Input: part model. Units: mm. Frame: model coordinates. A direction names the side the tool comes from. Round coordinates to 2 decimals unless told otherwise and drop trailing zeros. Order: outer loops, then holes, each group sorted by start corner. A loop starts at its lowest first (then second) coordinate and runs counter-clockwise, first axis right, second up. Notation, with made-up numbers: (68.5, 5.25) -> (114.5, 5.25) arc R24 ccw to (114.5, 16.25) -> close; hole circle Ø3 at (5.5, 35). An arc over 180 degrees is marked (long way). Use a Markdown table: item, result.
from build123d import *

# Parameters (mm, degrees)
SKETCH1_R           = 2.5
SKETCH1_R_2         = 1.3
BOSS_EXTRUDE1_DEPTH = 5
SKETCH2_W           = 40
SKETCH2_H           = 25
BOSS_EXTRUDE2_DEPTH = 10
SKETCH3_W           = 23
SKETCH3_H           = 13
CUT_EXTRUDE1_DEPTH  = 8
SKETCH3_3_R         = 1.05
CUT_EXTRUDE2_DEPTH  = 8
SKETCH3_4_W         = 23
SKETCH3_4_H         = 13
CUT_EXTRUDE3_DEPTH  = 11
FILLET1_R           = 10
CUT_EXTRUDE4_DEPTH  = 41


with BuildPart() as part:
    # Sketch1 → Boss-Extrude1 (new body)
    with BuildSketch(Plane(origin=(0, 0, 0), x_dir=(1, 0, 0), z_dir=(0, 1, 0))):
        with BuildLine():
            Line((0, 15), (25, 15))
            Line((25, 15), (25, -15))
            Line((25, -15), (0, -15))
            ThreePointArc((0, -15), (-15, 0), (0, 15))
        make_face()
        Circle(SKETCH1_R, mode=Mode.SUBTRACT)
        with Locations((0, -4.5)):
            Circle(SKETCH1_R_2, mode=Mode.SUBTRACT)
        with Locations((0, 4.5)):
            Circle(SKETCH1_R_2, mode=Mode.SUBTRACT)
    extrude(amount=BOSS_EXTRUDE1_DEPTH)

    # Sketch2 → Boss-Extrude2 (add)
    with BuildSketch(Plane(origin=(25, 0, 0), x_dir=(0, 0, -1), z_dir=(1, 0, 0))):
        with Locations((5, 12.5)):
            Rectangle(SKETCH2_W, SKETCH2_H)
    extrude(amount=BOSS_EXTRUDE2_DEPTH)

    # Sketch3 → Cut-Extrude1 (cut)
    with BuildSketch(Plane(origin=(25, 0, 0), x_dir=(0, 0, -1), z_dir=(1, 0, 0))):
        with Locations((5, 13)):
            Rectangle(SKETCH3_W, SKETCH3_H)
    extrude(amount=CUT_EXTRUDE1_DEPTH, mode=Mode.SUBTRACT)

    # Sketch3<3> → Cut-Extrude2 (cut)
    with BuildSketch(Plane(origin=(25, 0, 0), x_dir=(0, 0, -1), z_dir=(1, 0, 0))):
        with Locations((-9, 13)):
            Circle(SKETCH3_3_R)
        with Locations((19, 13)):
            Circle(SKETCH3_3_R)
    extrude(amount=CUT_EXTRUDE2_DEPTH, mode=Mode.SUBTRACT)

    # Sketch3<4> → Cut-Extrude3 (cut, through all)
    with BuildSketch(Plane(origin=(25, 0, 0), x_dir=(0, 0, -1), z_dir=(1, 0, 0))):
        with Locations((5, 13)):
            Rectangle(SKETCH3_4_W, SKETCH3_4_H)
    extrude(amount=CUT_EXTRUDE3_DEPTH, mode=Mode.SUBTRACT)

    # Fillet1
    fillet1_edges = [part.edges().sort_by_distance(p)[0] for p in [
        (30, 0, -25),
        (30, 25, -25),
        (30, 25, 15),
    ]]
    fillet(fillet1_edges, radius=FILLET1_R)

    # Sketch4 → Cut-Extrude4 (cut, through all)
    with BuildSketch(Plane.XY.offset(15)):
        Polygon((7, 0), (4, 3), (-4, 3), (-7, 0), align=None)
    extrude(amount=-CUT_EXTRUDE4_DEPTH, mode=Mode.SUBTRACT)


solid = part.part
1) Cut plane C-C on x = -9. Return loops of the section in (y, z).
Results found:
| item | result |
|---|---|
| outline | (0, -12) -> (5, -12) -> (5, 12) -> (0, 12) -> close |
2) Cut plane A-A on z = 0. Return loops of the section in (x, y), and give its area (3 significant figures).
Results found:
| item | result |
|---|---|
| outline | (-15, 0) -> (-7, 0) -> (-4, 3) -> (-2.5, 3) -> (-2.5, 5) -> (-15, 5) -> close; (2.5, 3) -> (4, 3) -> (7, 0) -> (35, 0) -> (35, 6.5) -> (25, 6.5) -> (25, 5) -> (2.5, 5) -> close; (25, 19.5) -> (35, 19.5) -> (35, 25) -> (25, 25) -> close |
| area | 277 mm² |
3) Line query: L1, parallel to Z at x = 0, y = 3.7; L2, parallel to Y at x = 11, z = 0.5; L3, parallel to X at y = 5.25, z = -13. Output: solid intervals per line, ascending. Write a range as [from, to].
Results found:
| item | result |
|---|---|
| L1 | z = [-15, -5.8], [-3.2, -2.5], [2.5, 3.2], [5.8, 15] |
| L2 | y = [0, 5] |
| L3 | x = [25, 35] |
4) Cut plane B-B on y = 13. Return loops of the section in (x, z).
Results found:
| item | result |
|---|---|
| outline | (25, -25) -> (35, -25) -> (35, -16.5) -> (25, -16.5) -> (25, -17.95) -> (33, -17.95) -> (33, -20.05) -> (25, -20.05) -> close; (25, 6.5) -> (35, 6.5) -> (35, 15) -> (25, 15) -> (25, 10.05) -> (33, 10.05) -> (33, 7.95) -> (25, 7.95) -> close |
5) Cut plane D-D on z = -19. Return loops of the section in (x, y), and give its area (3 significant figures).
Results found:
| item | result |
|---|---|
| outline | (25, 0.83) -> (35, 0.83) -> (35, 24.17) -> (25, 24.17) -> (25, 14.05) -> (33, 14.05) -> (33, 11.95) -> (25, 11.95) -> close |
| area | 217 mm² |
6) Set-up query: faces 5 (the flat face through (5, 5, 0)), 6 (the flat face through (-5, 2, 0)), 7 (the flat face through (30, 6.5, -5)), 8 (the flat face through (33, 13, 9)). Return all of +Z, -Z, +X, -X, +Y, -Y with unobstructed straight access to the full face (end or side cutting, diameter ignored); none if empty.
Results found:
| item | result |
|---|---|
| face 5 | +Z, -Z, -X, +Y |
| face 6 | +Z, -Z, -Y |
| face 7 | +X, -X |
| face 8 | -X |
7) Pull-direction query (Z, two-part tool) for faces 1 (the cylindrical face through (28.94, 13.05, -17.95)), 2 (the flat face through (21, 0, 0)), 3 (the cylindrical face through (-0.28, 3.99, -3.23)), 4 (the flat face through (12, 2, -15)); classes: +Z half, -Z half, draft (parallel to the pull), parting line (faces both ways), or undercut.
Results found:
| item | result |
|---|---|
| face 1 | undercut |
| face 2 | draft |
| face 3 | undercut |
| face 4 | -Z half |
8) Pin query (flat end, axial travel): pin 1 Ø1 at (x, z) = (12.5, -16) entering from -Y; pin 2 Ø0.6 at (y, z) = (12.5, -19) entering from -X; pin 3 Ø2.5 at (x, y) = (13, 3.5) entering from -Z; pin 4 Ø9 at (x, z) = (-2, 0.5) entering from -Y. Return the tip coordinate at first contact, or that it passes through.
Results found:
| item | result |
|---|---|
| pin 1 | passes through |
| pin 2 | stops at x = 33 |
| pin 3 | stops at z = -15 |
| pin 4 | stops at y = 0.5 |
